from build123d import *

# Parameters (mm, degrees)
M14X1_5_TAPPED_HOLE1_D              = 12.5
M14X1_5_TAPPED_HOLE1_DEPTH          = 25.4
M14X1_5_TAPPED_HOLE1_TIP            = 3.755378869
F_1_16_0_0625_DIAMETER_HOLE1_D      = 1.5875
F_1_16_0_0625_DIAMETER_HOLE1_DEPTH  = 28.575
F_1_16_0_0625_DIAMETER_HOLE1_TIP    = 0.476933116
F_3_32_0_09375_DIAMETER_HOLE1_D     = 2.38125
F_3_32_0_09375_DIAMETER_HOLE1_DEPTH = 28.702
F_3_32_0_09375_DIAMETER_HOLE1_TIP   = 0.715399675
F_1_4_CLEARANCE_HOLE1_D             = 6.7564
CIRPATTERN1_COUNT                   = 6
F_1_32_0_03125_DIAMETER_HOLE1_D     = 0.79375
F_1_32_0_03125_DIAMETER_HOLE1_DEPTH = 28.575
F_1_32_0_03125_DIAMETER_HOLE1_TIP   = 0.238466558
F_1_8_0_125_DIAMETER_HOLE1_D        = 3.175
F_1_8_0_125_DIAMETER_HOLE1_DEPTH    = 25.4
F_1_8_0_125_DIAMETER_HOLE1_TIP      = 0.953866233


with BuildPart() as part:
    # Sketch1 → Revolve1 (revolve)
    with BuildSketch(Plane.XY):
        Polygon((-20.6375, 0), (-31.75, 0), (-31.75, 38.1), (-3.556, 38.1), (-3.556, 6.35), (-4.7625, 6.35), (-11.1125, 0), (-17.5895, 0), (-17.5895, 2.032), (-20.6375, 2.032), align=None)
    revolve(axis=Axis((0, 0, 0), (0, 1, 0)))

    # M14x1.5 Tapped Hole1
    with Locations(Plane(origin=(0, 38.1, 0), x_dir=(1, 0, 0), z_dir=(0, 1, 0))):
        with Locations((0, 0)):
            Hole(M14X1_5_TAPPED_HOLE1_D / 2, depth=M14X1_5_TAPPED_HOLE1_DEPTH)
            with Locations((0, 0, -(M14X1_5_TAPPED_HOLE1_DEPTH + M14X1_5_TAPPED_HOLE1_TIP / 2))):  # 118° drill point
                Cone(0, M14X1_5_TAPPED_HOLE1_D / 2, M14X1_5_TAPPED_HOLE1_TIP, mode=Mode.SUBTRACT)

    # Sketch6 → 1_4 NPT Tapped Hole1 (revolve, cut)
    with BuildSketch(Plane(origin=(31.75, 19.05, 0), x_dir=(0, 0, -1), z_dir=(0, 1, 0))):
        Polygon((0, 0), (0, 20.360347279), (5.5626, 17.018), (5.5626, 9.906), (5.943685794, 9.906), (6.2402847, 0), align=None)
    revolve(axis=Axis((38.1, 19.05, 0), (-1, 0, 0)), mode=Mode.SUBTRACT)

    # Sketch8 → 1_4 NPT Tapped Hole2 (revolve, cut)
    with BuildSketch(Plane(origin=(-31.75, 19.05, 0), x_dir=(0, 0, 1), z_dir=(0, 1, 0))):
        Polygon((0, 0), (0, 20.360347279), (5.5626, 17.018), (5.5626, 9.906), (5.943685794, 9.906), (6.2402847, 0), align=None)
    revolve(axis=Axis((-38.1, 19.05, 0), (1, 0, 0)), mode=Mode.SUBTRACT)

    # 1_16 _0.0625_ Diameter Hole1
    with Locations(Plane(origin=(31.75, 0, 0), x_dir=(0, 0, -1), z_dir=(1, 0, 0))):
        with Locations((0, 19.05)):
            Hole(F_1_16_0_0625_DIAMETER_HOLE1_D / 2, depth=F_1_16_0_0625_DIAMETER_HOLE1_DEPTH)
            with Locations((0, 0, -(F_1_16_0_0625_DIAMETER_HOLE1_DEPTH + F_1_16_0_0625_DIAMETER_HOLE1_TIP / 2))):  # 118° drill point
                Cone(0, F_1_16_0_0625_DIAMETER_HOLE1_D / 2, F_1_16_0_0625_DIAMETER_HOLE1_TIP, mode=Mode.SUBTRACT)

    # 3_32 _0.09375_ Diameter Hole1
    with Locations(Plane.ZY.offset(31.75)):
        with Locations((0, 19.05)):
            Hole(F_3_32_0_09375_DIAMETER_HOLE1_D / 2, depth=F_3_32_0_09375_DIAMETER_HOLE1_DEPTH)
            with Locations((0, 0, -(F_3_32_0_09375_DIAMETER_HOLE1_DEPTH + F_3_32_0_09375_DIAMETER_HOLE1_TIP / 2))):  # 118° drill point
                Cone(0, F_3_32_0_09375_DIAMETER_HOLE1_D / 2, F_3_32_0_09375_DIAMETER_HOLE1_TIP, mode=Mode.SUBTRACT)

    # 1_4 Clearance Hole1 (through all)
    with Locations(Plane(origin=(0, 38.1, 0), x_dir=(1, 0, 0), z_dir=(0, 1, 0))):
        with Locations((21.997045256, 12.7)):
            f_1_4_clearance_hole1 = Hole(F_1_4_CLEARANCE_HOLE1_D / 2)

    # CirPattern1: 1_4 Clearance Hole1 ×6 about axis
    cirpattern1_axis = Axis((0, 0, 0), (0, 1, 0))
    for i in range(1, CIRPATTERN1_COUNT):
        add(f_1_4_clearance_hole1.rotate(cirpattern1_axis, i * 360 / CIRPATTERN1_COUNT), mode=Mode.SUBTRACT)

    # Sketch18 → 1_4 NPT Tapped Hole3 (revolve, cut)
    with BuildSketch(Plane(origin=(15.875, 19.05, -27.49630657), x_dir=(-0.866025404, 0, -0.5), z_dir=(0, 1, 0))):
        Polygon((0, 0), (0, 20.360347279), (5.5626, 17.018), (5.5626, 9.906), (5.943685794, 9.906), (6.2402847, 0), align=None)
    revolve(axis=Axis((19.05, 19.05, -32.995567884), (-0.5, 0, 0.866025404)), mode=Mode.SUBTRACT)

    # 1_32 _0.03125_ Diameter Hole1
    with Locations(Plane(origin=(15.875, 0, -27.49630657), x_dir=(0, -1, 0), z_dir=(0.5, 0, -0.866025404))):
        with Locations((-19.05, 0)):
            Hole(F_1_32_0_03125_DIAMETER_HOLE1_D / 2, depth=F_1_32_0_03125_DIAMETER_HOLE1_DEPTH)
            with Locations((0, 0, -(F_1_32_0_03125_DIAMETER_HOLE1_DEPTH + F_1_32_0_03125_DIAMETER_HOLE1_TIP / 2))):  # 118° drill point
                Cone(0, F_1_32_0_03125_DIAMETER_HOLE1_D / 2, F_1_32_0_03125_DIAMETER_HOLE1_TIP, mode=Mode.SUBTRACT)

    # 1_8 _0.125_ Diameter Hole1
    with Locations(Plane(origin=(0, 0, 0), x_dir=(0, 0, 1), z_dir=(0.707106781, -0.707106781, 0))):
        with Locations((0, 3.175)):
            Hole(F_1_8_0_125_DIAMETER_HOLE1_D / 2, depth=F_1_8_0_125_DIAMETER_HOLE1_DEPTH)
            with Locations((0, 0, -(F_1_8_0_125_DIAMETER_HOLE1_DEPTH + F_1_8_0_125_DIAMETER_HOLE1_TIP / 2))):  # 118° drill point
                Cone(0, F_1_8_0_125_DIAMETER_HOLE1_D / 2, F_1_8_0_125_DIAMETER_HOLE1_TIP, mode=Mode.SUBTRACT)


solid = part.part
Geometry check sheet. Reference: the model listing, model coordinates, mm. A direction names the side the tool comes from. Give positions to 0.01 mm unless a question says otherwise; leave off trailing zeros. Write each loop counter-clockwise with the first axis right and the second up, starting at its lowest first coordinate (ties: lowest second). Pieces come first, ordered by that corner, then holes. Notation, with made-up numbers: (-14.5, 75.25) - (38.5, 75.25) arc R7 ccw to (38.5, 80.25) - close; hole circle Ø6 at (38, -12.75). An arc over 180 degrees is marked (long way). Put each result on its own line as item: value.
1. Go/stop test with flat-tipped pins: pin 1 (10 mm diameter, centred on x = 0, z = 0, fed in from -Y); pin 2 (6 mm diameter, centred on x = -22, z = -12.7, fed in from -Y); pin 3 (8 mm diameter, centred on y = 29, z = 11, fed in from +X); pin 4 (8 mm diameter, centred on x = 21, y = 28.5, fed in from +Z). Record where each tip stops, or that it passes through.
Ans:
pin 1: stops at y = 6.11
pin 2: passes through
pin 3: stops at x = 30.97
pin 4: stops at z = 26.82
2. Sectioned sample at A-A, the plane z = 25.4. Enter the section's corners in (x, y).
Ans:
outline: (-19.05, 0) - (-3.38, 0) - (-3.38, 38.1) - (-19.05, 38.1) - close; (3.38, 0) - (19.05, 0) - (19.05, 38.1) - (3.38, 38.1) - close
3. Sectioned sample at B-B, the plane z = 12.7. Enter the section's corners in (x, y), plus the area to 3 significant figures.
Ans:
outline: (-29.1, 0) - (-25.38, 0) - (-25.38, 38.1) - (-29.1, 38.1) - close; (-18.62, 0) - (-16.27, 0) - (-16.27, 2.03) - (-12.17, 2.03) - (-12.17, 0) - (12.17, 0) - (12.17, 2.03) - (16.27, 2.03) - (16.27, 0) - (18.62, 0) - (18.62, 38.1) - (-18.62, 38.1) - close; (25.38, 0) - (29.1, 0) - (29.1, 38.1) - (25.38, 38.1) - close
area: 1,690 mm²
4. Sectioned sample at C-C, the plane z = -12.7. Give the number of separate pieces and of enclosed holes in the cut face, plus the area to 3 significant figures.
Ans:
separate pieces: 3
enclosed holes: 1
area: 1,610 mm²
5. Draft check along Y on faces 1 (the flat face through (15.2, 2.032, 9.3)), 2 (the conical face through (-26.87, 18.78, -6.09)), 3 (the conical face through (-0.807, 11.183, 3.636)). Enter one of: +Y half, -Y half, draft (parallel to the pull), parting line (faces both ways), or undercut.
Ans:
face 1: -Y half
face 2: undercut
face 3: +Y half
6. Set-up check for faces 4 (the cylindrical face through (-18.34, 24.48, -1.21)), 5 (the flat face through (-4, 6.35, 0)), 6 (the cylindrical face through (18.338, 17.379, -5.306)), 7 (the cylindrical face through (4.6, 19.4, -7.6)): record each of +Z, -Z, +X, -X, +Y, -Y from which the full face is reachable in a straight line by a thin tool's end or side.
Ans:
face 4: -X
face 5: -Y
face 6: +X
face 7: none
7. Thickness scan on line 1 (Z direction, x = 0, y = 9); line 2 (Z direction, x = 0, y = 18.5); line 3 (Z direction, x = -22, y = 5.5). Record the ranges inside material, lowest first.
Ans:
line 1: z = -31.75 to -28.78, -22.02 to -3.56, 3.56 to 22.02, 28.78 to 31.75
line 2: z = -31.75 to -28.78, -22.02 to -6.25, 6.25 to 22.02, 28.78 to 31.75
line 3: z = -22.89 to -16.08, -9.32 to 9.32, 16.08 to 22.89
